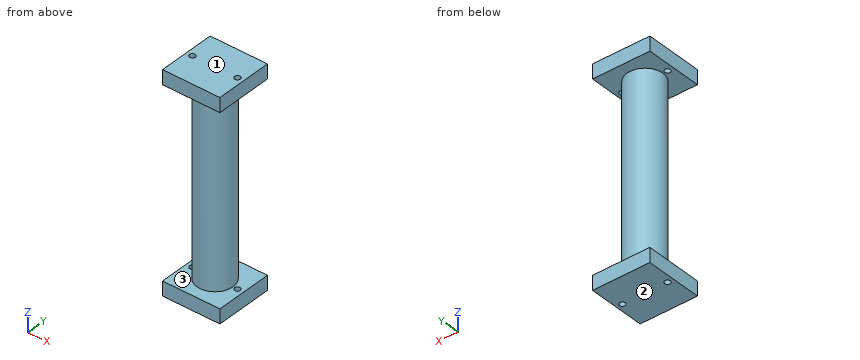
```python
from build123d import *

# Parameters (mm, degrees)
SKETCH_1_W          = 40
SKETCH_1_H          = 40
EXTRUDE_1_DEPTH     = 10
SKETCH_2_R          = 12.5
EXTRUDE_2_DEPTH     = 130
SKETCH_3_W          = 40
SKETCH_3_H          = 40
EXTRUDE_3_DEPTH     = 10
SKETCH_4_R          = 2
CUT_EXTRUDE_1_DEPTH = 10
SKETCH_5_R          = 2
CUT_EXTRUDE_2_DEPTH = 10
CUT_EXTRUDE_START   = -10
SKETCH_6_R          = 2
CUT_EXTRUDE_3_DEPTH = 10
SKETCH_7_R          = 2
CUT_EXTRUDE_4_DEPTH = 10


with BuildPart() as part:
    # 草圖1 → 填料-伸長1 (new body)
    with BuildSketch(Plane.XY):
        Rectangle(SKETCH_1_W, SKETCH_1_H)
    extrude(amount=EXTRUDE_1_DEPTH)

    # 草圖2 → 填料-伸長2 (add)
    with BuildSketch(Plane.XY.offset(10)):
        Circle(SKETCH_2_R)
    extrude(amount=EXTRUDE_2_DEPTH)

    # 草圖3 → 填料-伸長3 (add)
    with BuildSketch(Plane.XY.offset(140)):
        Rectangle(SKETCH_3_W, SKETCH_3_H)
    extrude(amount=EXTRUDE_3_DEPTH)

    # 草圖4 → 除料-伸長1 (cut)
    with BuildSketch(Plane.XY.offset(150)):
        with Locations((-15.713957528, 0)):
            Circle(SKETCH_4_R)
    extrude(amount=-CUT_EXTRUDE_1_DEPTH, mode=Mode.SUBTRACT)

    # 草圖5 → 除料-伸長2 (cut)
    with BuildSketch(Plane.XY.offset(150)):
        with Locations((15.71, 0)):
            Circle(SKETCH_5_R)
    extrude(amount=-CUT_EXTRUDE_2_DEPTH, mode=Mode.SUBTRACT)

    # 草圖6 → 除料-伸長3 (cut)
    with BuildSketch(Plane(origin=(0, 0, 0), x_dir=(-1, 0, 0), z_dir=(0, 0, -1)).offset(CUT_EXTRUDE_START)):
        with Locations(Location((-15.71, 0, 0), (0, 0, 180))):
            Circle(SKETCH_6_R)
    extrude(amount=CUT_EXTRUDE_3_DEPTH, mode=Mode.SUBTRACT)

    # 草圖7 → 除料-伸長4 (cut)
    with BuildSketch(Plane(origin=(0, 0, 0), x_dir=(-1, 0, 0), z_dir=(0, 0, -1))):
        with Locations((15.71, 0)):
            Circle(SKETCH_7_R)
    extrude(amount=-CUT_EXTRUDE_4_DEPTH, mode=Mode.SUBTRACT)


solid = part.part
```
The model under review builds one solid part; all positions refer to its coordinate system, in mm. Face numbers are marked on the shaded views. Round coordinates to 2 decimals unless told otherwise and drop trailing zeros. Loops run counter-clockwise (first coordinate to the right, second up) from the corner with the lowest first, then second, coordinate; pieces in that order, holes last.
Item 1: Take a section at B-B (x = 15.71). Write out the cut boundary in (y, z), then the cut area to 3 significant figures.
Determined:
outline: (-20, 0) - (-2, 0) - (-2, 10) - (-20, 10) - close; (-20, 140) - (-2, 140) - (-2, 150) - (-20, 150) - close; (2, 0) - (20, 0) - (20, 10) - (2, 10) - close; (2, 140) - (20, 140) - (20, 150) - (2, 150) - close
area: 720 mm2
Item 2: For line 1 (Z direction, x = -18, y = -16); line 2 (Y direction, x = 0, z = 27); line 3 (Y direction, x = 9, z = 139.5), list the stretches that pass through material, from the lowest coordinate up.
Determined:
line 1: z = 0 to 10, 140 to 150
line 2: y = -12.5 to 12.5
line 3: y = -8.67 to 8.67
Item 3: Take a section at C-C (y = 0). Write out the cut boundary in (x, z).
Determined:
outline: (-20, 0) - (-17.71, 0) - (-17.71, 10) - (-20, 10) - close; (-20, 140) - (-17.71, 140) - (-17.71, 150) - (-20, 150) - close; (-13.71, 0) - (13.71, 0) - (13.71, 10) - (12.5, 10) - (12.5, 140) - (13.71, 140) - (13.71, 150) - (-13.71, 150) - (-13.71, 140) - (-12.5, 140) - (-12.5, 10) - (-13.71, 10) - close; (17.71, 0) - (20, 0) - (20, 10) - (17.71, 10) - close; (17.71, 140) - (20, 140) - (20, 150) - (17.71, 150) - close
Item 4: Take a section at A-A (y = 17.5). Write out the cut boundary in (x, z), then the cut area to 3 significant figures.
Determined:
outline: (-20, 0) - (20, 0) - (20, 10) - (-20, 10) - close; (-20, 140) - (20, 140) - (20, 150) - (-20, 150) - close
area: 800 mm2
Item 5: Take a section at D-D (x = 0). Write out the cut boundary in (y, z), then the cut area to 3 significant figures.
Determined:
outline: (-20, 0) - (20, 0) - (20, 10) - (12.5, 10) - (12.5, 140) - (20, 140) - (20, 150) - (-20, 150) - (-20, 140) - (-12.5, 140) - (-12.5, 10) - (-20, 10) - close
area: 4,050 mm2
Item 6: Mouldability with a two-part tool opening along Z and no side actions: class the marked faces 1, 2 and 3 as released by +Z, released by -Z, zero draft, split by the parting line, or undercut.
Determined:
face 1: released by +Z
face 2: released by -Z
face 3: undercut
Item 7: Clearance check with flat-ended pins moving along their axes: pin 1 Ø8 at (y, z) = (-11.5, 67.5) entering from +X; pin 2 Ø12 at (x, z) = (-5.5, 59) entering from +Y; pin 3 Ø2 at (x, z) = (0.5, 42.5) entering from -Y; pin 4 Ø3.5 at (x, y) = (-15.71, 0) entering from +Z. State where each tip first meets the part, or that it passes through.
Determined:
pin 1: stops at x = 10
pin 2: stops at y = 12.5
pin 3: stops at y = -12.5
pin 4: passes through
